Geometry check sheet. Reference: the model listing, model coordinates, mm. Face numbers are marked on the shaded views. A direction names the side the tool comes from. Coordinates: 2 decimals unless noted, no trailing zeros. Order: outer loops, then holes, each group sorted by start corner. A loop starts at its lowest first (then second) coordinate and runs counter-clockwise, first axis right, second up. Notation, with made-up numbers: (48, 7.25) - (99, 7.25) arc R24 ccw to (99, 27.25) - close; hole circle Ø3 at (-10.75, 21.5). An arc over 180 degrees is marked (long way). Use CSV: the item, a comma, the result in double quotes. Start each with the question number.
1) Tool access check on the marked faces 1 and 2. Record the directions out of +Z, -Z, +X, -X, +Y, -Y that give a thin tool (end or side, any length) a straight path to the whole face; none if there is none.
2) Sectioned sample at C-C, the plane z = 9. Record the cut outline in (x, y).
3) Thickness scan on probe 1 along Z at (x, y) = (-4.5, 2); probe 2 along Y at (x, z) = (2.5, -7.5); probe 3 along Y at (x, z) = (3.5, 0). Record the ranges inside material, lowest first. Write a range as [from, to].
4) Depth check by flat-ended pin: P1, Ø2, axis at x = -2.5, z = -5, coming from the +Y side; P2, Ø2, axis at y = -3.5, z = 1.5, coming from the -X side; P3, Ø2, axis at x = 3, y = 2, coming from the -Z side; P4, Ø5, axis at x = 3, z = 9, coming from the -Y side. Enter the tip coordinate at first touch or a pass-through.
from build123d import *

# Parameters (mm, degrees)
SKETCH1_R           = 4
BOSS_EXTRUDE1_DEPTH = 15
SKETCH2_R           = 6
BOSS_EXTRUDE2_DEPTH = 3
FILLET1_R           = 1


with BuildPart() as part:
    # Sketch1 → Boss-Extrude1 (new, symmetric)
    with BuildSketch(Plane.XY):
        Circle(SKETCH1_R)
    extrude(amount=BOSS_EXTRUDE1_DEPTH, both=True)

    # Sketch2 → Boss-Extrude2 (add)
    with BuildSketch(Plane.XY.offset(15)):
        Circle(SKETCH2_R)
    extrude(amount=BOSS_EXTRUDE2_DEPTH)

    # Fillet1
    fillet1_edges = [part.edges().sort_by_distance(p)[0] for p in [
        (-4, 0, -15),
        (-4, 0, 15),
        (-6, 0, 15),
        (-6, 0, 18),
    ]]
    fillet(fillet1_edges, radius=FILLET1_R - 0.0001)  # a hair under: the kernel refuses the full size


solid = part.part
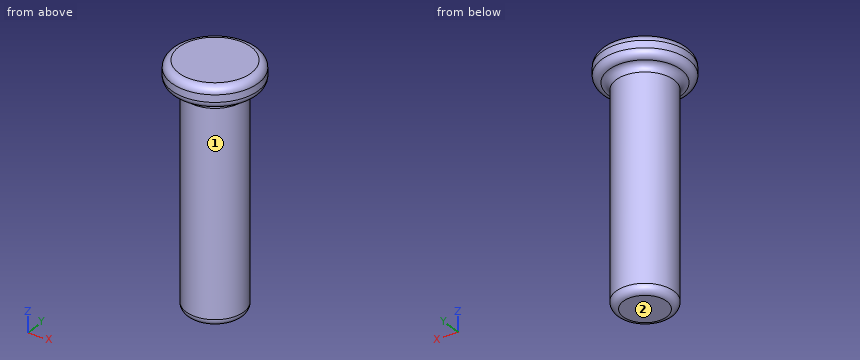
Evaluation:
1,face 1,"-Z"
1,face 2,"-Z, +X, -X, +Y, -Y"
2,outline,"circle Ø8 at (0, 0)"
3,probe 1,"[15, 18]"
3,probe 2,"[-3.12, 3.12]"
3,probe 3,"[-1.94, 1.94]"
4,P1,"y = 3.71"
4,P2,"x = -3.12"
4,P3,"z = -15"
4,P4,"y = -3.97"
